Can you work these out from the model? Positions are in its coordinate system, mm. Face numbers are marked on the shaded views. A direction names the side the tool comes from. Give positions to 0.01 mm unless a question says otherwise; leave off trailing zeros. Order: outer loops, then holes, each group sorted by start corner. A loop starts at its lowest first (then second) coordinate and runs counter-clockwise, first axis right, second up.
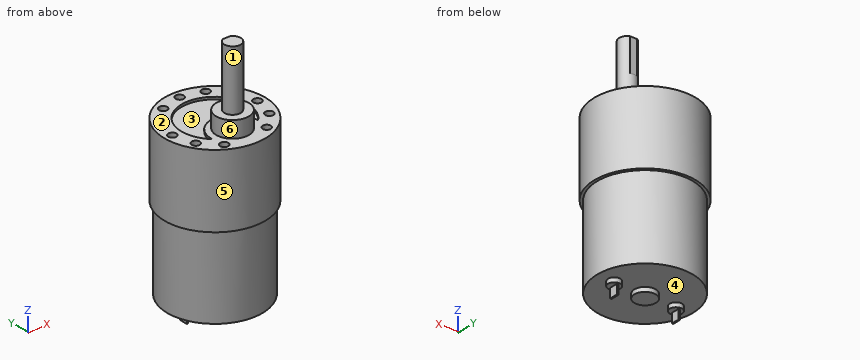
```python
from build123d import *

# Parameters (mm, degrees)
CROQUIS1_R              = 18.4
SALIENTE_EXTRUIR1_DEPTH = 26.5
CORTAR_EXTRUIR2_DEPTH   = 0.85
CROQUIS3_R              = 1.5
CORTAR_EXTRUIR3_DEPTH   = 25
CROQUIS9_R              = 1.5
CORTAR_EXTRUIR4_DEPTH   = 5
CROQUIS22_R             = 6
SALIENTE_EXTRUIR2_DEPTH = 6
CROQUIS24_R             = 3
SALIENTE_EXTRUIR3_DEPTH = 22
CORTAR_EXTRUIR5_DEPTH   = 12
CROQUIS26_R             = 17.4
SALIENTE_EXTRUIR4_DEPTH = 30
CROQUIS27_R             = 3.9
CROQUIS27_R_2           = 2.25
CROQUIS27_W             = 0.5
CROQUIS27_H             = 3
SALIENTE_EXTRUIR5_DEPTH = 1.6
CROQUIS29_W             = 0.5
CROQUIS29_H             = 3
SALIENTE_EXTRUIR6_DEPTH = 5


with BuildPart() as part:
    # Croquis1 → Saliente-Extruir1 (new body)
    with BuildSketch(Plane.XY):
        Circle(CROQUIS1_R)
    extrude(amount=SALIENTE_EXTRUIR1_DEPTH)

    # Croquis2 → Cortar-Extruir2 (cut)
    with BuildSketch(Plane.XY.offset(26.5)):
        with BuildLine():
            ThreePointArc((8.4190219, -8.8295), (-0.043589152, 12.19992213), (-8.355713846, -8.889434523))
            ThreePointArc((-8.355713846, -8.889434523), (0, 0), (8.4190219, -8.8295))
        make_face()
    extrude(amount=-CORTAR_EXTRUIR2_DEPTH, mode=Mode.SUBTRACT)

    # Croquis3 → Cortar-Extruir3 (cut)
    with BuildSketch(Plane.XY.offset(26.5)):
        with Locations((0, 15.5)):
            Circle(CROQUIS3_R)
        with Locations((13.423393759, -7.75)):
            Circle(CROQUIS3_R)
        with Locations((-13.423393759, -7.75)):
            Circle(CROQUIS3_R)
    extrude(amount=-CORTAR_EXTRUIR3_DEPTH, mode=Mode.SUBTRACT)

    # Croquis9 → Cortar-Extruir4 (cut)
    with BuildSketch(Plane.XY.offset(26.5)):
        with Locations((-15.5, 0)):
            Circle(CROQUIS9_R)
        with Locations((-7.75, 13.423393759)):
            Circle(CROQUIS9_R)
        with Locations((7.75, 13.423393759)):
            Circle(CROQUIS9_R)
        with Locations((15.5, 0)):
            Circle(CROQUIS9_R)
        with Locations((7.75, -13.423393759)):
            Circle(CROQUIS9_R)
        with Locations((-7.75, -13.423393759)):
            Circle(CROQUIS9_R)
    extrude(amount=-CORTAR_EXTRUIR4_DEPTH, mode=Mode.SUBTRACT)

    # Croquis22 → Saliente-Extruir2 (add)
    with BuildSketch(Plane.XY.offset(26.5)):
        with Locations((0, -7.75)):
            Circle(CROQUIS22_R)
    extrude(amount=SALIENTE_EXTRUIR2_DEPTH)

    # Croquis24 → Saliente-Extruir3 (add)
    with BuildSketch(Plane.XY.offset(32.5)):
        with Locations((0, -7.75)):
            Circle(CROQUIS24_R)
    extrude(amount=SALIENTE_EXTRUIR3_DEPTH)

    # Croquis25 → Cortar-Extruir5 (cut)
    with BuildSketch(Plane.XY.offset(54.5)):
        Polygon((-72.570863995, -5.05), (-1.307669683, -5.05), (1.307669683, -5.05), (72.570863995, -5.05), (72.570863995, 137.476388625), (-72.570863995, 137.476388625), align=None)
    extrude(amount=-CORTAR_EXTRUIR5_DEPTH, mode=Mode.SUBTRACT)

    # Croquis26 → Saliente-Extruir4 (add)
    with BuildSketch(Plane(origin=(0, 0, 0), x_dir=(-1, 0, 0), z_dir=(0, 0, -1))):
        Circle(CROQUIS26_R)
    extrude(amount=SALIENTE_EXTRUIR4_DEPTH)

    # Croquis27 → Saliente-Extruir5 (add)
    with BuildSketch(Plane(origin=(0, 0, -30), x_dir=(-1, 0, 0), z_dir=(0, 0, -1))):
        Circle(CROQUIS27_R)
        with Locations((-11.25, 0)):
            Circle(CROQUIS27_R_2)
        with Locations((-11.25, 0)):
            Rectangle(CROQUIS27_W, CROQUIS27_H, mode=Mode.SUBTRACT)
        with Locations((11.25, 0)):
            Circle(CROQUIS27_R_2)
        with Locations((11.25, 0)):
            Rectangle(CROQUIS27_W, CROQUIS27_H, mode=Mode.SUBTRACT)
    extrude(amount=SALIENTE_EXTRUIR5_DEPTH)

    # Croquis29 → Saliente-Extruir6 (add)
    with BuildSketch(Plane(origin=(0, 0, -30), x_dir=(-1, 0, 0), z_dir=(0, 0, -1))):
        with Locations((-11.25, 0)):
            Rectangle(CROQUIS29_W, CROQUIS29_H)
        with Locations((11.25, 0)):
            Rectangle(CROQUIS29_W, CROQUIS29_H)
    extrude(amount=SALIENTE_EXTRUIR6_DEPTH)


solid = part.part
```
1) We'd pull the mould along X, two halves only. Please class the marked faces 1, 2 and 3: +X half, -X half, draft (parallel to the pull), parting line (faces both ways), or undercut.
2) I'm going to push flat-ended pins straight in: pin 1 Ø1.8 at (x, y) = (-15.5, 0) entering from -Z; pin 2 Ø3.5 at (x, y) = (-7.5, 13.5) entering from +Z; pin 3 Ø1.5 at (x, y) = (-13.5, -7.5) entering from +Z. Where does each tip first touch, or does it pass through?
3) Suppose I cut it at B-B (z = 8.5). Please give me the cut outline in (x, y).
4) If I drill on line 1 (X direction, y = -7, z = 19); line 2 (Y direction, x = -7.75, z = 22.95); line 3 (Z direction, x = -4.5, y = -9), over which ranges is the centre line in solid material (lowest first)?
5) Suppose I cut it at D-D (z = 34). Please give me the cut outline in (x, y), and give its area (3 significant figures).
6) Which directions (+Z, -Z, +X, -X, +Y, -Y) give clear straight access to the entire face, cutting with the end or side of a thin tool? Please do the marked faces 4, 5 and 6.
7) Suppose I cut it at C-C (y = 7.5). Please give me the cut outline in (x, z).
Results:
1. face 1: parting line
1. face 2: draft
1. face 3: undercut
2. pin 1: stops at z = -30
2. pin 2: stops at z = 26.5
2. pin 3: stops at z = 1.5
3. outline: circle Ø36.8 at (0, 0); hole circle Ø3 at (-13.42, -7.75); hole circle Ø3 at (0, 15.5); hole circle Ø3 at (13.42, -7.75)
4. line 1: x = -17.02 to -14.72, -12.12 to 12.12, 14.72 to 17.02
4. line 2: y = -16.69 to -14.92, -11.92 to 11.92, 14.92 to 16.69
4. line 3: z = -30 to 32.5
5. outline: circle Ø6 at (0, -7.75)
5. area: 28.3 mm2
6. face 4: -Z
6. face 5: +Z, -Z
6. face 6: +Z
7. outline: (-16.8, 0) - (-15.7, 0) - (-15.7, -30) - (15.7, -30) - (15.7, 0) - (16.8, 0) - (16.8, 26.5) - (9.62, 26.5) - (9.62, 25.65) - (-9.62, 25.65) - (-9.62, 26.5) - (-16.8, 26.5) - close
